Design review of the part built by this model. Coordinates are the model's own, in mm. Face numbers are marked on the shaded views. A direction names the side the tool comes from. Coordinates: 2 decimals unless noted, no trailing zeros. Order: outer loops, then holes, each group sorted by start corner. A loop starts at its lowest first (then second) coordinate and runs counter-clockwise, first axis right, second up.
from build123d import *

# Parameters (mm, degrees)
F1_DEPTH = 76.2
F0_W     = 22.0843532517
F0_H     = 12.7000030306
F2_DEPTH = 25.4
F4_DEPTH = 6.35


# Not quite as in the source:
# - the program builds the solid bodies; features that only make, move or delete a surface that nothing else refers to are left out


with BuildPart() as f1:
    # F0 (on Front) → F1 (new body, symmetric)
    with BuildSketch(Plane.XZ):
        Polygon((30.5117662821, 21.1660526693), (-33.6534492671, 21.1660526693), (-33.6534492671, -27.1129291505), (43.2117693126, -27.1129291505), (43.2117693126, 21.1660526693), align=None)
    extrude(amount=F1_DEPTH, both=True)

    # F0 (on Front) → F2 (join, symmetric)
    with BuildSketch(Plane.XZ):
        with Locations((102.8505478717, 75.5138860928)):
            Rectangle(F0_W, F0_H)
        with BuildLine():
            Line((30.5117662821, 36.1293591958), (30.5117662821, 21.1660526693))
            Line((30.5117662821, 21.1660526693), (43.2117693126, 21.1660526693))
            Line((43.2117693126, 21.1660526693), (43.2117693126, 36.1293591958))
            ThreePointArc((43.2117693126, 36.1293591958), (52.8873577836, 59.4882961065), (76.2462946943, 69.1638845775))
            Line((76.2462946943, 69.1638845775), (91.8083712459, 69.1638845775))
            Line((91.8083712459, 69.1638845775), (91.8083712459, 81.8638876081))
            Line((91.8083712459, 81.8638876081), (76.2462946943, 81.8638876081))
            ThreePointArc((76.2462946943, 81.8638876081), (43.9070995196, 68.4685543705), (30.5117662821, 36.1293591958))
        make_face()
    extrude(amount=F2_DEPTH, both=True)

    # F0 (on Front) → F4 (join, symmetric)
    with BuildSketch(Plane.XZ):
        with BuildLine():
            add(Edge.make_bspline(
                [(-33.6534492671, 21.1660526693), (-9.9662784487, 49.1574853659), (15.5614716932, 83.2813158631), (76.2462946943, 81.8638876081)],
                knots=[0, 0, 0, 0, 125.5475244242, 125.5475244242, 125.5475244242, 125.5475244242], degree=3))
            Line((-33.6534492671, 21.1660526693), (30.5117662821, 21.1660526693))
            Line((30.5117662821, 21.1660526693), (30.5117662821, 36.1293591958))
            ThreePointArc((30.5117662821, 36.1293591958), (43.9070995196, 68.4685543705), (76.2462946943, 81.8638876081))
        make_face()
    extrude(amount=F4_DEPTH, both=True)

    # F0 (on Front) → F5 (revolve)
    with BuildSketch(Plane.XZ):
        Polygon((113.8927244975, 100.2546474338), (113.8927244975, 81.8638876081), (113.8927244975, 69.1638845775), (113.8927244975, 64.6806582808), (139.1344815493, 64.6806582808), (139.1344815493, 100.2546474338), align=None)
    revolve(axis=Axis((113.8927244975, 0, 84.7092660056), (0, 0, 1)))


solid = f1.part
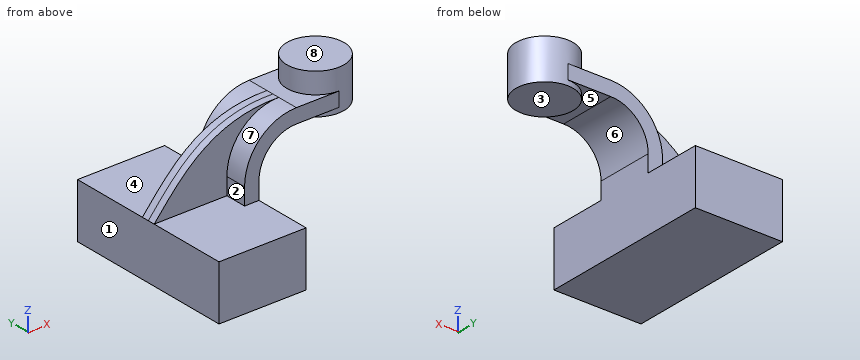
1. To check wall thickness, follow line 1 (Z direction, x = -23, y = -34.5); line 2 (X direction, y = 53.5, z = -1); line 3 (X direction, y = -14, z = 29.5). State the ranges of each line that lie inside material, in increasing order.
2. Insertion check: pin 1 (1.5 mm diameter, centred on x = 23.5, y = 24.5, fed in from +Z); pin 2 (4.5 mm diameter, centred on y = -19, z = 30, fed in from -X); pin 3 (6 mm diameter, centred on y = -21, z = 64.5, fed in from -X). Each pin has a flat end and moves straight along its axis. Give the tip position at first contact, or say it passes through.
3. Add section B-B (z = 8). Give the boundary of the cut face in (x, y).
4. Add section A-A (y = 37). Give the boundary of the cut face in (x, z).
5. For the marked faces 1, 2, 3 and 4, list the 3-axis set-ups (+Z, -Z, +X, -X, +Y, -Y) from which the entire face can be reached by the end or side of a thin tool; tool diameter is ignored.
6. Mouldability with a two-part tool opening along X and no side actions: class the marked faces 5, 6, 7 and 8 as pulls with the +X half, pulls with the -X half, needs draft (parallel to the pull), parting line crosses it, or undercut.
Solution:
1. line 1: z = -27.11 to 21.17
1. line 2: x = -33.65 to 43.21
1. line 3: x = 30.51 to 43.21
2. pin 1: stops at z = 21.17
2. pin 2: stops at x = 30.51
2. pin 3: stops at x = 38.19
3. outline: (-33.65, -76.2) - (43.21, -76.2) - (43.21, 76.2) - (-33.65, 76.2) - close
4. outline: (-33.65, -27.11) - (43.21, -27.11) - (43.21, 21.17) - (-33.65, 21.17) - close
5. face 1: +Z, -Z, -X, +Y, -Y
5. face 2: +Z, -X, -Y
5. face 3: -Z, +X, +Y, -Y
5. face 4: +Z, -X, +Y
6. face 5: undercut
6. face 6: undercut
6. face 7: pulls with the -X half
6. face 8: needs draft
